Model file for the job. Use its own axes, mm. Face numbers are marked on the shaded views. A direction names the side the tool comes from. Coordinates: 2 decimals unless noted, no trailing zeros. Order: outer loops, then holes, each group sorted by start corner. A loop starts at its lowest first (then second) coordinate and runs counter-clockwise, first axis right, second up. Notation, with made-up numbers: (-17, 47.5) -> (5, 47.5) arc R34 cw to (5, 86.5) -> close; hole circle Ø7 at (6, -35.75). An arc over 180 degrees is marked (long way). Use CSV: the item, a comma, the result in double quotes. Start each with the question number.
(1) Pull direction Y, two halves, no side cores. Call the marked faces 4, 5, 6 and 7: pulls with the +Y half, pulls with the -Y half, needs draft (parallel to the pull), parting line crosses it, or undercut.
(2) Cut at B-B on y = -38. Write the cut outline in (x, z), plus the area to 3 significant figures.
(3) Cut at C-C on z = 12.5. Give the number of separate pieces and of enclosed holes in the cut face, plus the area to 3 significant figures.
(4) Probe L1, parallel to Y at x = 0, z = 22.75; L2, parallel to Z at x = -31.5, y = -30; L3, parallel to X at y = -23.25, z = 23.9. List the from-to ranges inside material, lowest first.
(5) Tool access for the marked faces 1, 2 and 3: list every direction of +Z, -Z, +X, -X, +Y, -Y with a clear straight run to the whole face (end or side of a thin tool).
(6) Cut at A-A on x = -20.5. Write the cut outline in (y, z).
(7) Pin check, flat tips, straight feed: pin 1 Ø3.5 at (x, y) = (-39.5, 23) entering from -Z; pin 2 Ø2 at (x, z) = (-8, 11.5) entering from +Y; pin 3 Ø8 at (y, z) = (-16.5, 9.5) entering from +X; pin 4 Ø6 at (y, z) = (24.5, 10) entering from +X. Stop position of each tip, or through.
```python
from build123d import *

# Parameters (mm, degrees)
SKETCH_1_R               = 49.5
SKETCH_1_R_2             = 43
SKETCH_1_R_3             = 1.75
EXTRUDE_1_DEPTH          = 25
CUT_EXTRUDE_1_DEPTH      = 59
PATTERN_CIRCULAR_1_COUNT = 6
SKETCH_3_R               = 44.045845484
EXTRUDE_2_DEPTH          = 3
CUT_EXTRUDE_3_DEPTH      = 22


with BuildPart() as part:
    # Эскиз1 → Бобышка-Вытянуть1 (new body)
    with BuildSketch(Plane.XY):
        Circle(SKETCH_1_R)
        Circle(SKETCH_1_R_2, mode=Mode.SUBTRACT)
        with Locations((0, 46.5)):
            Circle(SKETCH_1_R_3, mode=Mode.SUBTRACT)
        with Locations((40.270181276, 23.25)):
            Circle(SKETCH_1_R_3, mode=Mode.SUBTRACT)
        with Locations((40.270181276, -23.25)):
            Circle(SKETCH_1_R_3, mode=Mode.SUBTRACT)
        with Locations((0, -46.5)):
            Circle(SKETCH_1_R_3, mode=Mode.SUBTRACT)
        with Locations((-40.270181276, -23.25)):
            Circle(SKETCH_1_R_3, mode=Mode.SUBTRACT)
        with Locations((-40.270181276, 23.25)):
            Circle(SKETCH_1_R_3, mode=Mode.SUBTRACT)
    extrude(amount=EXTRUDE_1_DEPTH)

    # Эскиз2 → Вырез-Вытянуть1 (cut)
    with BuildSketch(Plane(origin=(0, 0, 0), x_dir=(0, 0, -1), z_dir=(1, 0, 0))):
        with BuildLine():
            Line((-5, 12.5), (-5, -12.5))
            ThreePointArc((-5, -12.5), (-12.5, -20), (-20, -12.5))
            Line((-20, -12.5), (-20, 12.5))
            ThreePointArc((-20, 12.5), (-12.5, 20), (-5, 12.5))
        make_face()
    cut_extrude_1 = extrude(amount=-CUT_EXTRUDE_1_DEPTH, mode=Mode.SUBTRACT)

    # Круговой массив1: Вырез-Вытянуть1 ×6 about axis
    pattern_circular_1_axis = Axis((0, 0, 25), (0, 0, -1))
    for i in range(1, PATTERN_CIRCULAR_1_COUNT):
        add(cut_extrude_1.rotate(pattern_circular_1_axis, i * 360 / PATTERN_CIRCULAR_1_COUNT), mode=Mode.SUBTRACT)

    # Эскиз3 → Бобышка-Вытянуть2 (add)
    with BuildSketch(Plane(origin=(0, 0, 0), x_dir=(-1, 0, 0), z_dir=(0, 0, -1))):
        Circle(SKETCH_3_R)
    extrude(amount=-EXTRUDE_2_DEPTH)

    # Эскиз4 → Вырез-Вытянуть3 (cut)
    with BuildSketch(Plane(origin=(0, 0, 0), x_dir=(-1, 0, 0), z_dir=(0, 0, -1))):
        with BuildLine():
            Line((-3, 46.5), (-3, 53.502718932))
            ThreePointArc((-3, 53.502718932), (0, 56.502718932), (3, 53.502718932))
            Line((3, 53.502718932), (3, 46.5))
            ThreePointArc((3, 46.5), (0, 43.5), (-3, 46.5))
        make_face()
        with BuildLine():
            Line((-41.770181276, 20.651923789), (-47.834713767, 24.153283255))
            ThreePointArc((-47.834713767, 24.153283255), (-48.932789978, 28.251359466), (-44.834713767, 29.349435677))
            Line((-44.834713767, 29.349435677), (-38.770181276, 25.848076211))
            ThreePointArc((-38.770181276, 25.848076211), (-37.672105065, 21.75), (-41.770181276, 20.651923789))
        make_face()
        with BuildLine():
            Line((-38.770181276, -25.848076211), (-44.834713767, -29.349435677))
            ThreePointArc((-44.834713767, -29.349435677), (-48.932789978, -28.251359466), (-47.834713767, -24.153283255))
            Line((-47.834713767, -24.153283255), (-41.770181276, -20.651923789))
            ThreePointArc((-41.770181276, -20.651923789), (-37.672105065, -21.75), (-38.770181276, -25.848076211))
        make_face()
        with BuildLine():
            Line((3, -46.5), (3, -53.502718932))
            ThreePointArc((3, -53.502718932), (0, -56.502718932), (-3, -53.502718932))
            Line((-3, -53.502718932), (-3, -46.5))
            ThreePointArc((-3, -46.5), (0, -43.5), (3, -46.5))
        make_face()
        with BuildLine():
            Line((41.770181276, -20.651923789), (47.834713767, -24.153283255))
            ThreePointArc((47.834713767, -24.153283255), (48.932789978, -28.251359466), (44.834713767, -29.349435677))
            Line((44.834713767, -29.349435677), (38.770181276, -25.848076211))
            ThreePointArc((38.770181276, -25.848076211), (37.672105065, -21.75), (41.770181276, -20.651923789))
        make_face()
        with BuildLine():
            Line((38.770181276, 25.848076211), (44.834713767, 29.349435677))
            ThreePointArc((44.834713767, 29.349435677), (48.932789978, 28.251359466), (47.834713767, 24.153283255))
            Line((47.834713767, 24.153283255), (41.770181276, 20.651923789))
            ThreePointArc((41.770181276, 20.651923789), (37.672105065, 21.75), (38.770181276, 25.848076211))
        make_face()
    extrude(amount=-CUT_EXTRUDE_3_DEPTH, mode=Mode.SUBTRACT)


solid = part.part
```
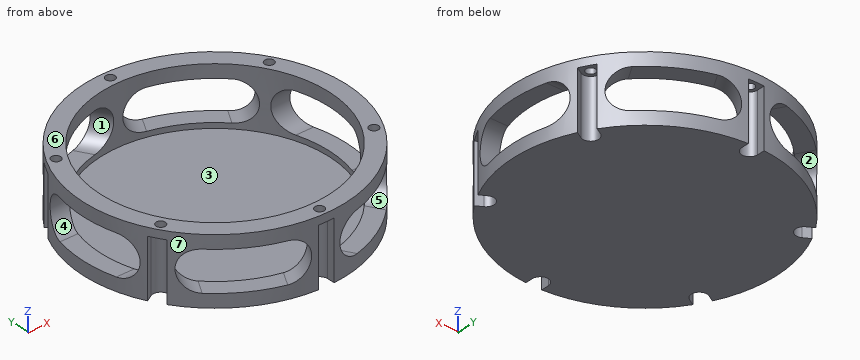
Outcome:
1,face 4,"undercut"
1,face 5,"pulls with the -Y half"
1,face 6,"needs draft"
1,face 7,"parting line crosses it"
2,outline,"(-31.72, 0) -> (31.72, 0) -> (31.72, 5) -> (20.12, 5) -> (20.12, 3) -> (-20.12, 3) -> (-20.12, 5) -> (-31.72, 5) -> close; (-31.72, 20) -> (-20.12, 20) -> (-20.12, 25) -> (-31.72, 25) -> close; (20.12, 20) -> (31.72, 20) -> (31.72, 25) -> (20.12, 25) -> close"
2,area,"353 mm2"
3,separate pieces,"6"
3,enclosed holes,"0"
3,area,"83.6 mm2"
4,L1,"-49.5 to -48.25, -44.75 to -43, 43 to 44.75, 48.25 to 49.5"
4,L2,"0 to 5, 20 to 25"
4,L3,"-43.7 to -42.02, -38.52 to -36.17, 36.17 to 38.52, 42.02 to 43.7"
5,face 1,"-X"
5,face 2,"+Y"
5,face 3,"+Z"
6,outline,"(-45.06, 0) -> (45.06, 0) -> (45.06, 5) -> (37.8, 5) -> (37.8, 3) -> (-37.8, 3) -> (-37.8, 5) -> (-45.06, 5) -> close; (-45.06, 20) -> (-37.8, 20) -> (-37.8, 25) -> (-45.06, 25) -> close; (37.8, 20) -> (45.06, 20) -> (45.06, 25) -> (37.8, 25) -> close"
7,pin 1,"z = 22"
7,pin 2,"through"
7,pin 3,"x = 47.01"
7,pin 4,"x = 44.59"
